Autodesk Inventor part; units mm, degrees
ref_plane "YZ Plane" through (0, 0, 0) normal (1, 0, 0) x (0, 1, 0)
ref_plane "XZ Plane" through (0, 0, 0) normal (0, 1, 0) x (-1, 0, 0)
ref_plane "XY Plane" through (0, 0, 0) normal (0, 0, 1) x (1, 0, 0)
sketch "Sketch1" plane through (0, 0, 0) normal (0, 1, 0) x (-1, 0, 0)
  line L0 (0, 0) -> (-114.3, 0)
  line L1 (-114.3, 0) -> (-114.3, -146.05)
  line L2 (-114.3, -146.05) -> (0, -146.05)
  line L3 (0, -146.05) -> (0, 0)
  dimension "d0" = 114.3
  dimension "d1" = 146.05
extrude "Extrusion1" add sketch "Sketch1" against normal blind 6.35
sketch "Sketch2" plane through (0, 0, 0) normal (0, 1, 0) x (1, 0, 0)
  line L0 (-6.35, 151.892) -> (-6.35, -3.175)
  line L1 (0, 146.05) -> (0, 0)
  line L2 (-6.35, 151.892) -> (120.65, 151.892)
  line L3 (114.3, 146.05) -> (0, 146.05)
  line L4 (120.65, 151.892) -> (120.65, -3.175)
  line L5 (114.3, 0) -> (114.3, 146.05)
  line L6 (-6.35, -3.175) -> (120.65, -3.175)
  line L7 (0, 0) -> (114.3, 0)
  dimension "d5" = 6.35
  dimension "d6" = 5.842
  dimension "d7" = 6.35
  dimension "d8" = 3.175
extrude "Extrusion2" add sketch "Sketch2" along normal blind 6.35 contours L2 L4 L6 L0 | L3 L5 L7 L1
sketch "Sketch3" plane through (0, 6.35, 0) normal (0, 1, 0) x (1, 0, 0)
  line L0 (50.8, 113.792) -> (63.5, 113.792)
  line L1 (63.5, 113.792) -> (63.5, 102.362)
  line L2 (63.5, 102.362) -> (50.8, 102.362)
  line L3 (50.8, 102.362) -> (50.8, 113.792)
  circle A0 centre (42.545, 108.712) radius 1.5875
  circle A1 centre (71.755, 108.712) radius 1.5875
  line L4 (120.65, 151.892) -> (-6.35, 151.892)
  line L5 (-6.35, 151.892) -> (-6.35, -3.175)
  point P0 (0, 0)
  dimension "d11" = 12.7
  dimension "d12" = 11.43
  dimension "d13" = 3.175
  dimension "d14" = 3.175
  dimension "d15" = 8.255
  dimension "d16" = 8.255
  dimension "d19" = 38.1
  dimension "d20" = 57.15
  dimension "d21" = 6.35
  dimension "d22" = 6.35
extrude "Extrusion3" cut sketch "Sketch3" against normal blind 25.4
sketch "Sketch4" plane through (0, -6.35, 0) normal (0, -1, 0) x (1, 0, 0)
  line L0 (0, 0) -> (114.3, 0)
  line L1 (114.3, 0) -> (114.3, -146.05)
  line L2 (114.3, -146.05) -> (0, -146.05)
  line L3 (0, -146.05) -> (0, 0)
  line L4 (1.016, -1.016) -> (113.284, -1.016)
  line L5 (113.284, -1.016) -> (113.284, -145.034)
  line L6 (113.284, -145.034) -> (1.016, -145.034)
  line L7 (1.016, -145.034) -> (1.016, -1.016)
  dimension "d27" = 1.016
extrude "Extrusion4" cut sketch "Sketch4" against normal blind 6.35
shell "Shell1" thickness 2.54 removed faces 1 at (59.2667, -6.35, -34.798)
sketch "Sketch5" plane through (0, -6.35, 0) normal (0, -1, 0) x (1, 0, 0)
  circle A0 centre (71.755, -108.712) radius 1.5875
  circle A1 centre (71.755, -108.712) radius 4.1275
  circle A2 centre (42.545, -108.712) radius 1.5875
  circle A3 centre (42.545, -108.712) radius 4.1275
  line L0 (66.04, -99.822) -> (48.26, -99.822)
  line L1 (48.26, -99.822) -> (48.26, -116.332)
  line L2 (48.26, -116.332) -> (66.04, -116.332)
  line L3 (66.04, -116.332) -> (66.04, -99.822)
  point P0 (0, 0)
extrude "Extrusion5" cut sketch "Sketch5" against normal blind 10.3188
properties part number "button_angle_top"
Check sheet for the modelled part. Datum: model origin and axes. Units: mm. A direction names the side the tool comes from. Round coordinates to 2 decimals unless told otherwise and drop trailing zeros. Loops run counter-clockwise (first coordinate to the right, second up) from the corner with the lowest first, then second, coordinate; pieces in that order, holes last. Notation, with made-up numbers: (75, -28) - (128, -28) arc R33 ccw to (128, 5) - close; hole circle Ø10 at (27, 2). An arc over 180 degrees is marked (long way). Answer as a JSON object with one key per item and string values. Group by question number.
Q1. Gauge pin test, flat ends, axial feed: P1, Ø5, axis at x = 98.5, y = -3.5, coming from the +Z side; P2, Ø5, axis at x = 44.5, z = -35, coming from the -Y side; P3, Ø6.5, axis at x = 42.545, z = -108.712, coming from the -Y side. Record the tip position at first contact, or that the pin passes through.
Q2. Scan lines: line 1 along X through (y, z) = (-5.5, -63); line 2 along X through (y, z) = (3.5, -50); line 3 along Z through (x, y) = (67.5, -3.5). Record each from-to range of solid material in increasing order. Write a range as [from, to].
Q3. Mould release check, pull along Z, two halves, no side actions. Record for faces 1 (the face through (58, -2, -142.494)), 2 (the face through (1.016, -3, -74)), 3 (the face through (56, -3, -1.016)): released by +Z, released by -Z, zero draft, split by the parting line, or undercut.
Q4. Set-up check for faces 4 (the face through (113.284, -3, -72)), 5 (the face through (58, -3, -145.034)), 6 (the face through (57, 3.969, -101)), 7 (the face through (3, 2.54, -80)): record each of +Z, -Z, +X, -X, +Y, -Y from which the full face is reachable in a straight line by a thin tool's end or side.
Q5. Sectioned sample at C-C, the plane x = 104.5. Enter the section's corners in (y, z) (3 decimals), plus the area to 3 significant figures.
Q6. Sectioned sample at A-A, the plane y = -4.25. Enter the section's corners in (x, z), plus the area to 3 significant figures.
Q7. Sectioned sample at B-B, the plane z = -13. Enter the section's corners in (x, y), plus the area to 3 significant figures.
Solution:
{
 "1": {"P1": "stops at z = -1.02", "P2": "stops at y = 3.81", "P3": "stops at y = 3.97"},
 "2": {"line 1": "x = [1.02, 3.56], [110.74, 113.28]", "line 2": "x = [-6.35, -3.81], [118.11, 120.65]", "line 3": "z = [-145.03, -142.49], [-3.56, -1.02]"},
 "3": {"face 1": "undercut", "face 2": "zero draft", "face 3": "released by +Z"},
 "4": {"face 4": "+Z, -Z, +X, -Y", "face 5": "-Z, +X, -X, -Y", "face 6": "-Y", "face 7": "none"},
 "5": {"outline": "(-6.35, -145.034) - (0, -145.034) - (0, -151.892) - (6.35, -151.892) - (6.35, 3.175) - (0, 3.175) - (0, -1.016) - (-6.35, -1.016) - (-6.35, -3.556) - (2.54, -3.556) - (2.54, 0.635) - (3.81, 0.635) - (3.81, -149.352) - (2.54, -149.352) - (2.54, -142.494) - (-6.35, -142.494) - close", "area": "474 mm²"},
 "6": {"outline": "(1.02, -145.03) - (113.28, -145.03) - (113.28, -1.02) - (1.02, -1.02) - close; hole (3.56, -142.49) - (110.74, -142.49) - (110.74, -3.56) - (3.56, -3.56) - close", "area": "1,280 mm²"},
 "7": {"outline": "(-6.35, 0) - (1.02, 0) - (1.02, -6.35) - (3.56, -6.35) - (3.56, 2.54) - (-3.81, 2.54) - (-3.81, 3.81) - (118.11, 3.81) - (118.11, 2.54) - (110.74, 2.54) - (110.74, -6.35) - (113.28, -6.35) - (113.28, 0) - (120.65, 0) - (120.65, 6.35) - (-6.35, 6.35) - close", "area": "412 mm²"}
}
